Autodesk Inventor part; units mm, degrees
ref_plane "YZ Plane" through (0, 0, 0) normal (1, 0, 0) x (0, 1, 0)
ref_plane "XZ Plane" through (0, 0, 0) normal (0, 1, 0) x (-1, 0, 0)
ref_plane "XY Plane" through (0, 0, 0) normal (0, 0, 1) x (1, 0, 0)
sketch "Skizze1" plane through (0, 0, 0) normal (0, 0, 1) x (1, 0, 0)
  line L0 (-65, 0) -> (65, 0)
  line L1 (65, 0) -> (65, 20)
  line L2 (65, 20) -> (40, 20)
  line L3 (40, 20) -> (40, 54)
  line L4 (-65, 41) -> (-65, 0)
  line L5 (-65, 41) -> (-65, 41)
  line L6 (-65, 54) -> (-65, 54)
  line L7 (-65, 54) -> (-65, 41)
  line L8 (24, 71) -> (24, 54)
  line L9 (24, 54) -> (40, 54)
  line L10 (-65, 54) -> (24, 54)
  line L11 (24, 54) -> (24, 57)
  line L12 (24, 57) -> (-65, 57)
  line L13 (-65, 57) -> (-65, 54)
  line L14 (24, 71) -> (-65, 71)
  line L15 (-65, 71) -> (-65, 54)
  line L16 (43, 23) -> (68, 23)
  line L17 (68, 23) -> (68, -3)
  line L18 (68, -3) -> (-68, -3)
  line L19 (-68, -3) -> (-68, 44)
  line L20 (-68, 44) -> (-68, 44)
  line L21 (-68, 44) -> (-68, 57)
  line L22 (-68, 57) -> (-68, 57)
  line L23 (-68, 57) -> (-68, 74)
  line L24 (-68, 74) -> (27, 74)
  line L25 (27, 74) -> (27, 57)
  line L26 (27, 57) -> (43, 57)
  line L27 (43, 57) -> (43, 23)
  line L28 (-65, 71) -> (-51, 71)
  line L29 (-51, 71) -> (-51, 66)
  line L30 (-51, 66) -> (-65, 66)
  line L31 (-65, 66) -> (-65, 71)
  line L32 (8, 71) -> (-8, 71)
  line L33 (-8, 71) -> (-8, 66)
  line L34 (-8, 66) -> (8, 66)
  line L35 (8, 66) -> (8, 71)
  line L36 (-65, 71) -> (-55, 71)
  line L37 (-55, 71) -> (-55, 66)
  line L38 (-55, 66) -> (-65, 66)
  line L39 (-65, 66) -> (-65, 71)
  line L40 (1, 71) -> (-4, 71)
  line L41 (-4, 71) -> (-4, 66)
  line L42 (-4, 66) -> (1, 66)
  line L43 (1, 66) -> (1, 71)
  line L44 (8, 71) -> (1, 71)
  line L45 (1, 71) -> (1, 66)
  line L46 (1, 66) -> (8, 66)
  line L47 (8, 66) -> (8, 71)
  line L48 (-4, 71) -> (-8, 71)
  line L49 (-8, 71) -> (-8, 66)
  line L50 (-8, 66) -> (-4, 66)
  line L51 (-4, 66) -> (-4, 71)
  line L52 (8, 57) -> (-8, 57)
  line L53 (-8, 57) -> (-8, 60.5)
  line L54 (-8, 60.5) -> (8, 60.5)
  line L55 (8, 60.5) -> (8, 57)
  line L56 (1, 60.5) -> (-4, 60.5)
  line L57 (-4, 60.5) -> (-4, 57)
  line L58 (-4, 57) -> (1, 57)
  line L59 (1, 57) -> (1, 60.5)
  line L60 (-65, 57) -> (-51, 57)
  line L61 (-51, 57) -> (-51, 60.5)
  line L62 (-51, 60.5) -> (-65, 60.5)
  line L63 (-65, 60.5) -> (-65, 57)
  line L64 (-55, 60.5) -> (-65, 60.5)
  line L65 (-65, 60.5) -> (-65, 57)
  line L66 (-65, 57) -> (-55, 57)
  line L67 (-55, 57) -> (-55, 60.5)
  line L68 (-65, 57) -> (24, 57)
  line L69 (24, 57) -> (24, 54)
  line L70 (24, 54) -> (-65, 54)
  line L71 (-65, 54) -> (-65, 57)
  point P0 (0, 0)
  point P1 (0, 0)
  point P2 (0, 0)
  point P3 (0, 0)
  dimension "d0" = 130
  dimension "d1" = 25
  dimension "d2" = 20
  dimension "d3" = 41
  dimension "d4" = 54
  dimension "d16" = 0
  dimension "d17" = 89
  dimension "d18" = 71
  dimension "d19" = 3
  dimension "d21" = 16
  dimension "d22" = 14
  dimension "d23" = 5
  dimension "d24" = 43
  dimension "d25" = 10
  dimension "d26" = 51
  dimension "d27" = 5
  dimension "d28" = 5.5
  dimension "d31" = 3
  dimension "d41" = 0
extrude "Extrusion1" add sketch "Skizze1" against normal blind 3 contours L4 L7 L10 L9 L3 L2 L1 L0 | L13 L12 L8 L10 | L15 L62 L67 L12 | L12 L55 L54 L53 L61 L62 L15 L30 L29 L14 L33 L34 L35 L8 | L67 L62 L61 L12 | L12 L59 L54 L55 | L15 L14 L37 L30 | L35 L34 L43 L14 | L12 L57 L54 L59 | L53 L54 L57 L12 | L37 L14 L29 L30 | L43 L34 L41 L14 | L41 L34 L33 L14 | L16 L17 L18 L19 L21 L23 L24 L25 L26 L27
extrude "Extrusion2" add sketch "Skizze1" along normal blind 62 contours L13 L12 L8 L10 | L15 L62 L67 L12 | L67 L62 L61 L12 | L12 L59 L54 L55 | L15 L14 L37 L30 | L35 L34 L43 L14 | L12 L57 L54 L59 | L53 L54 L57 L12 | L37 L14 L29 L30 | L43 L34 L41 L14 | L41 L34 L33 L14 | L16 L17 L18 L19 L21 L23 L24 L25 L26 L27
sketch "Skizze2" plane through (-68, 74, -3) normal (0, 1, 0) x (1, 0, 0)
  line L0 (95, -65) -> (95, 0)
  line L1 (95, -65) -> (0, -65)
  line L2 (92, -65) -> (76, -65)
  arc A0 (88.5, -65) -> (77, -65) centre (82.75, -66.7139) ccw
  line L3 (77, -65) -> (88.5, -65)
  point P0 (68, -3)
  dimension "d36" = 6
  dimension "d37" = 12.25
  dimension "d38" = 11.5
extrude "Extrusion3" cut sketch "Skizze2" against normal up to surface (3 mm away)
properties part number "Erweiterung"
Geometry check sheet. Reference: the model listing, model coordinates, mm. A direction names the side the tool comes from. Round coordinates to 2 decimals unless told otherwise and drop trailing zeros. Loops run counter-clockwise (first coordinate to the right, second up) from the corner with the lowest first, then second, coordinate; pieces in that order, holes last. Notation, with made-up numbers: M -5,49.25 L 26,49.25 A33 cw 26,81.25 Z; hole C 10,11.5 d4. An arc over 180 degrees is marked long. Return JSON: item names as keys, results as strings. Group by question number.
(1) Go/stop test with flat-tipped pins: pin 1 (3 mm diameter, centred on x = -27, y = 39.5, fed in from +Z); pin 2 (5 mm diameter, centred on y = 67, z = 25.5, fed in from +X); pin 3 (6 mm diameter, centred on y = 48.5, z = 6, fed in from +X). Record where each tip stops, or that it passes through.
(2) Section check A-A, the plane y = 69.5. Enter the section's corners in (x, z).
(3) Set-up check for faces 4 (the face through (14.858, 72.521, 57.715)), 5 (the face through (-16, 36, -3)), 6 (the face through (16, 71, 31)), 7 (the face through (-10, 56, 62)), 8 (the face through (55, 23, 29)): record each of +Z, -Z, +X, -X, +Y, -Y from which the full face is reachable in a straight line by a thin tool's end or side.
(4) Section check B-B, the plane z = 40. Give the number of separate pieces and of enclosed holes in the cut face, and give its area (3 significant figures).
(5) Section check D-D, the plane y = 28.5. Enter the section's corners in (x, z), and give its area (3 significant figures).
(6) Mould release check, pull along Y, two halves, no side actions. Record for faces 1 (the face through (-68, 35, 29)), 2 (the face through (40, 37, 31)), 3 (the face through (1, -3, 29)): pulls with the +Y half, pulls with the -Y half, needs draft (parallel to the pull), parting line crosses it, or undercut.
(7) Section check C-C, the plane x = -11. Enter the section's corners in (y, z).
(8) Scan lines: line 1 along Y through (x, z) = (-21, 52); line 2 along Y through (x, z) = (-59, 46.5); line 3 along Y through (x, z) = (44, 2). Record each from-to range of solid material in increasing order. Write a range as [from, to].
Data:
{
 "1": {"pin 1": "z = 0", "pin 2": "x = 27", "pin 3": "x = 43"},
 "2": {"outline": "M -68,-3 L 27,-3 L 27,62 L 24,62 L 24,0 L 8,0 L 8,62 L -8,62 L -8,0 L -51,0 L -51,62 L -68,62 Z"},
 "3": {"face 4": "+Z, +Y", "face 5": "-Z, +X, -X, +Y, -Y", "face 6": "+Z", "face 7": "+Z, +X, -X, +Y, -Y", "face 8": "+Z, -Z, +X, +Y"},
 "4": {"separate pieces": "1", "enclosed holes": "2", "area": "1,760 mm²"},
 "5": {"outline": "M -68,-3 L 43,-3 L 43,62 L 40,62 L 40,0 L -65,0 L -65,62 L -68,62 Z", "area": "705 mm²"},
 "6": {"face 1": "needs draft", "face 2": "undercut", "face 3": "pulls with the -Y half"},
 "7": {"outline": "M -3,-3 L 74,-3 L 74,62 L 71,62 L 71,0 L 57,0 L 57,62 L 54,62 L 54,0 L 0,0 L 0,62 L -3,62 Z"},
 "8": {"line 1": "[-3, 0], [54, 57], [71, 74]", "line 2": "[-3, 0], [54, 60.5], [66, 74]", "line 3": "[-3, 0], [20, 23]"}
}
